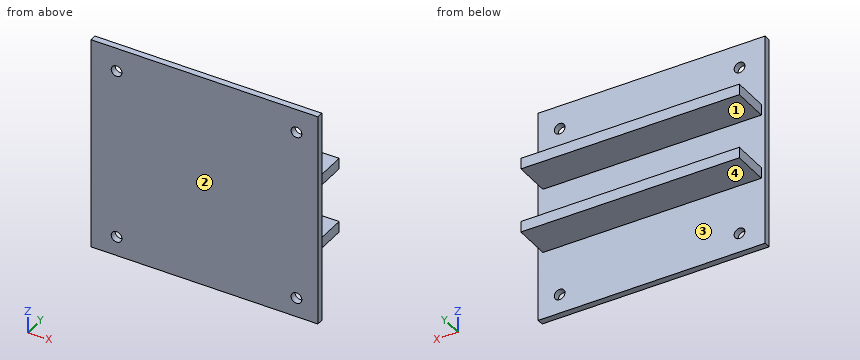
from build123d import *

# Parameters (mm, degrees)
SCHIZZO1_W                   = 53
SCHIZZO1_H                   = 50
ESTRUSIONE_ESTRUSIONE1_DEPTH = 1.5
SCHIZZO2_W                   = 51
SCHIZZO2_H                   = 2.54
ESTRUSIONE_ESTRUSIONE2_DEPTH = 8.5
SCHIZZO3_R                   = 1.25
TAGLIO_ESTRUSIONE1_DEPTH     = 8.5


with BuildPart() as part:
    # Schizzo1 → Estrusione-Estrusione1 (new body)
    with BuildSketch(Plane(origin=(0, 0, 0), x_dir=(1, 0, 0), z_dir=(0, 1, 0))):
        Rectangle(SCHIZZO1_W, SCHIZZO1_H)
    extrude(amount=ESTRUSIONE_ESTRUSIONE1_DEPTH)

    # Schizzo2 → Estrusione-Estrusione2 (add)
    with BuildSketch(Plane(origin=(0, 1.5, 0), x_dir=(1, 0, 0), z_dir=(0, 1, 0))):
        with Locations((-0.1, 7.73)):
            Rectangle(SCHIZZO2_W, SCHIZZO2_H)
        with Locations((-0.1, -7.51)):
            Rectangle(SCHIZZO2_W, SCHIZZO2_H)
    extrude(amount=ESTRUSIONE_ESTRUSIONE2_DEPTH)

    # Schizzo3 → Taglio-Estrusione1 (cut)
    with BuildSketch(Plane(origin=(0, 1.5, 0), x_dir=(1, 0, 0), z_dir=(0, 1, 0))):
        with Locations((21.5, 20.5)):
            Circle(SCHIZZO3_R)
        with Locations((-20.5, 20.5)):
            Circle(SCHIZZO3_R)
        with Locations((21.5, -19.5)):
            Circle(SCHIZZO3_R)
        with Locations((-20.5, -19.5)):
            Circle(SCHIZZO3_R)
    extrude(amount=-TAGLIO_ESTRUSIONE1_DEPTH, mode=Mode.SUBTRACT)


solid = part.part
Could you check a few things on this model? Use its own coordinates, in mm. Face numbers are marked on the shaded views. Give positions to 0.01 mm unless a question says otherwise; leave off trailing zeros. Order: outer loops, then holes, each group sorted by start corner. A loop starts at its lowest first (then second) coordinate and runs counter-clockwise, first axis right, second up.
1. We'd pull the mould along Z, two halves only. Please class the marked faces 1, 2, 3 and 4: pulls with the +Z half, pulls with the -Z half, needs draft (parallel to the pull), parting line crosses it, or undercut.
2. Suppose I cut it at C-C (y = 8.5). List the corners of the cut face in (x, z) for me.
3. Suppose I cut it at A-A (x = -20.5). List the corners of the cut face in (y, z) for me, plus the area to 3 significant figures.
4. Will these pins go through, and if not, where does the flat tip stop? P1, Ø2, axis at y = 3, z = -18.5, coming from the -X side; P2, Ø1.3, axis at y = 5, z = -8.5, coming from the +X side; P3, Ø3, axis at x = 21.5, z = 19.5, coming from the +Y side; P4, Ø2.5, axis at x = -11, y = 7, coming from the +Z side.
5. I need wall thicknesses on L1, parallel to Z at x = -20.5, y = 0.75; L2, parallel to X at y = 0.9, z = -20.5; L3, parallel to Z at x = 13.5, y = 9.25. Which ranges of each line are inside material? Lowest first, please.
6. Suppose I cut it at D-D (x = 18.5). List the corners of the cut face in (y, z) for me, plus the area to 3 significant figures.
7. Suppose I cut it at B-B (z = -20.5). List the corners of the cut face in (x, y) for me.
Solved:
1. face 1: undercut
1. face 2: needs draft
1. face 3: undercut
1. face 4: pulls with the -Z half
2. outline: (-25.6, -9) - (25.4, -9) - (25.4, -6.46) - (-25.6, -6.46) - close; (-25.6, 6.24) - (25.4, 6.24) - (25.4, 8.78) - (-25.6, 8.78) - close
3. outline: (0, -25) - (1.5, -25) - (1.5, -21.75) - (0, -21.75) - close; (0, -19.25) - (1.5, -19.25) - (1.5, -9) - (10, -9) - (10, -6.46) - (1.5, -6.46) - (1.5, 6.24) - (10, 6.24) - (10, 8.78) - (1.5, 8.78) - (1.5, 18.25) - (0, 18.25) - close; (0, 20.75) - (1.5, 20.75) - (1.5, 25) - (0, 25) - close
3. area: 111 mm2
4. P1: passes through
4. P2: stops at x = 25.4
4. P3: stops at y = 1.5
4. P4: stops at z = 8.78
5. L1: z = -25 to -21.75, -19.25 to 18.25, 20.75 to 25
5. L2: x = -26.5 to -21.75, -19.25 to 20.25, 22.75 to 26.5
5. L3: z = -9 to -6.46, 6.24 to 8.78
6. outline: (0, -25) - (1.5, -25) - (1.5, -9) - (10, -9) - (10, -6.46) - (1.5, -6.46) - (1.5, 6.24) - (10, 6.24) - (10, 8.78) - (1.5, 8.78) - (1.5, 25) - (0, 25) - close
6. area: 118 mm2
7. outline: (-26.5, 0) - (-21.75, 0) - (-21.75, 1.5) - (-26.5, 1.5) - close; (-19.25, 0) - (20.25, 0) - (20.25, 1.5) - (-19.25, 1.5) - close; (22.75, 0) - (26.5, 0) - (26.5, 1.5) - (22.75, 1.5) - close
